Source: CAD feature listing. Evaluate the final solid. Frame: model axes, mm. Face numbers are marked on the shaded views. A direction names the side the tool comes from. Round coordinates to 2 decimals unless told otherwise and drop trailing zeros. Write each loop counter-clockwise with the first axis right and the second up, starting at its lowest first coordinate (ties: lowest second). Pieces come first, ordered by that corner, then holes. Notation, with made-up numbers: (31.25, -37) -> (40.25, -37) arc R18 cw to (40.25, -17) -> close; hole circle Ø8 at (-20.75, 81.25). An arc over 180 degrees is marked (long way). Return JSON: item names as keys, results as strings. Group by question number.
from build123d import *

# Parameters (mm, degrees)
BOSS_EXTRUDE1_DEPTH = 5
FILLET1_R           = 5
FILLET3_R           = 1
FILLET4_R           = 1


with BuildPart() as part:
    # Sketch1 → Boss-Extrude1 (new body)
    with BuildSketch(Plane.XY):
        with BuildLine():
            Line((-1.7, 5.806246636), (-1.7, 1.145643924))
            ThreePointArc((-1.7, 1.145643924), (0, -2.05), (1.7, 1.145643924))
            Line((1.7, 1.145643924), (1.7, 5.806246636))
            ThreePointArc((1.7, 5.806246636), (0, -6.05), (-1.7, 5.806246636))
        make_face()
    extrude(amount=BOSS_EXTRUDE1_DEPTH)

    # Fillet1
    fillet1_edges = [part.edges().sort_by_distance(p)[0] for p in [
        (-1.7, 1.145643924, 2.5),
        (1.7, 1.145643924, 2.5),
    ]]
    fillet(fillet1_edges, radius=FILLET1_R)

    # Fillet3
    fillet3_edges = [part.edges().sort_by_distance(p)[0] for p in [
        (-1.7, 5.806246636, 2.5),
        (1.7, 5.806246636, 2.5),
    ]]
    fillet(fillet3_edges, radius=FILLET3_R)

    # Fillet4
    fillet4_edges = [part.edges().sort_by_distance(p)[0] for p in [
        (0, -2.05, 0),
        (0, -2.05, 5),
        (-1.7, 3.230675835, 0),
        (-1.762446697, 1.405980108, 0),
        (1.762446697, 1.405980108, 0),
        (-1.7, 3.230675835, 5),
        (-1.762446697, 1.405980108, 5),
        (1.762446697, 1.405980108, 5),
        (1.7, 3.230675835, 0),
        (1.7, 3.230675835, 5),
        (0, -6.05, 0),
        (-2.217637826, 5.143582452, 0),
        (2.217637826, 5.143582452, 0),
        (0, -6.05, 5),
        (-2.217637826, 5.143582452, 5),
        (2.217637826, 5.143582452, 5),
    ]]
    fillet(fillet4_edges, radius=FILLET4_R)


solid = part.part
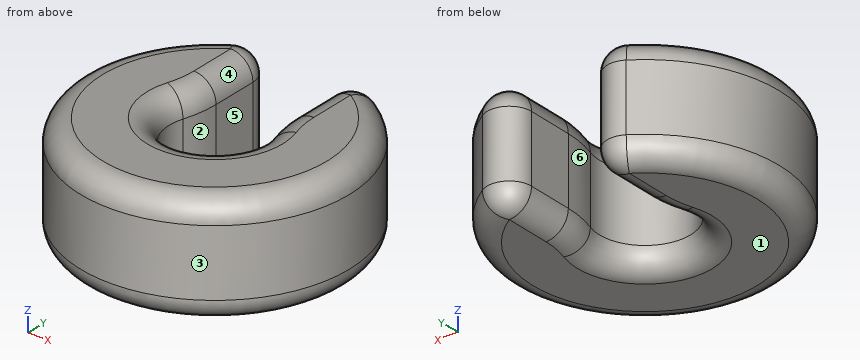
Item 1: Cut plane B-B on z = 2.45. Output: boundary loops of the cut face in (x, y), and give its area (3 significant figures).
Item 2: First-contact query: pin 1 Ø2.5 at (y, z) = (3.5, 3) entering from -X; pin 2 Ø2 at (x, z) = (-1.5, 2) entering from +Y; pin 3 Ø0.6 at (y, z) = (3.5, 3) entering from +X. Flat tips, straight axial feed; report the tip coordinate or a pass-through.
Item 3: Set-up query: the marked faces 4, 5 and 6. Return all of +Z, -Z, +X, -X, +Y, -Y with unobstructed straight access to the full face (end or side cutting, diameter ignored); none if empty.
Item 4: Pull-direction query (X, two-part tool) for the marked faces 1, 2 and 3; classes: +X half, -X half, draft (parallel to the pull), parting line (faces both ways), or undercut.
Item 5: Material intervals for probe 1 along X at (y, z) = (0, 2.6); probe 2 along Y at (x, z) = (0, 3.45); probe 3 along X at (y, z) = (3.75, 2.3), sorted ascending.
Item 6: Cut plane A-A on x = 0. Output: boundary loops of the cut face in (y, z).
Here are the results:
{
 "1": {"outline": "(-3.23, 5.11) arc R6.05 ccw (long way) to (3.23, 5.11) arc R1 ccw to (1.7, 4.27) -> (1.7, 2.19) arc R5 ccw to (1.95, 0.64) arc R2.05 cw (long way) to (-1.95, 0.64) arc R5 ccw to (-1.7, 2.19) -> (-1.7, 4.27) arc R1 ccw to start", "area": "86.2 mm^2"},
 "2": {"pin 1": "stops at x = -5.62", "pin 2": "stops at y = 5.25", "pin 3": "stops at x = 5.13"},
 "3": {"face 4": "+Z, +Y", "face 5": "+Z, -Z, +Y", "face 6": "+Z, -Z"},
 "4": {"face 1": "draft", "face 2": "undercut", "face 3": "parting line"},
 "5": {"probe 1": "x = -6.05 to -2.05, 2.05 to 6.05", "probe 2": "y = -6.05 to -2.05", "probe 3": "x = -4.75 to -1.7, 1.7 to 4.75"},
 "6": {"outline": "(-6.05, 1) arc R1 ccw to (-5.05, 0) -> (-3.05, 0) arc R1 ccw to (-2.05, 1) -> (-2.05, 4) arc R1 ccw to (-3.05, 5) -> (-5.05, 5) arc R1 ccw to (-6.05, 4) -> close"}
}
